For this review, use the dimensioned drawing (mm, ordinates from the lowest corner) and the shaded views. Round coordinates to 2 decimals unless told otherwise and drop trailing zeros. Loops run counter-clockwise (first coordinate to the right, second up) from the corner with the lowest first, then second, coordinate; pieces in that order, holes last.
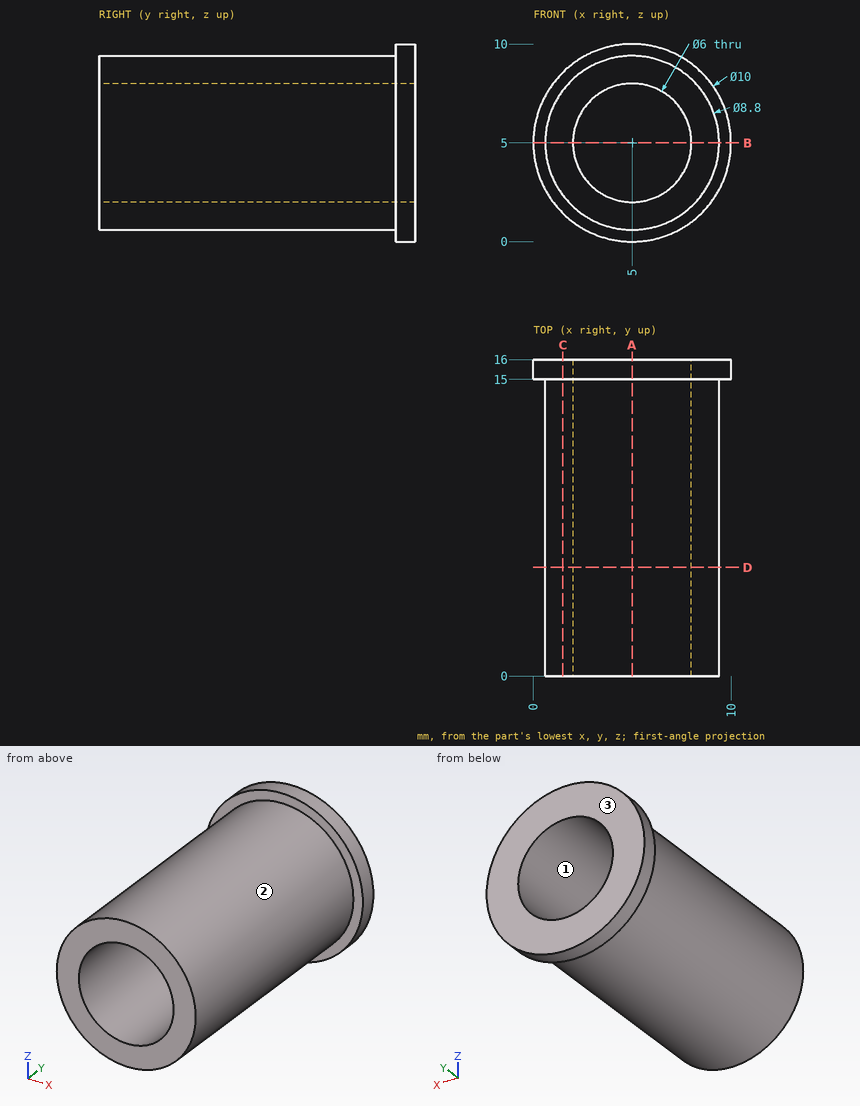
(1) Add section B-B (z = 5). Give the boundary of the cut face in (x, y).
(2) Insertion check: pin 1 Ø1 at (y, z) = (7.5, 1) entering from -X; pin 2 Ø3 at (x, y) = (7.5, 2) entering from +Z; pin 3 Ø4 at (x, y) = (1, 3) entering from +Z. Each pin has a flat end and moves straight along its axis. Give the tip position at first contact, or say it passes through.
(3) Add section D-D (y = 5.5). Give the boundary of the cut face in (x, z), plus the area to 3 significant figures.
(4) Add section C-C (x = 1.5). Give the boundary of the cut face in (y, z).
(5) For L1, parallel to Z at x = 5, y = 8; L2, parallel to Z at x = 3.25, y = 14; L3, parallel to Y at x = 6.75, z = 0.5, list the stretches that pass through material, from the lowest coordinate up.
(6) Add section A-A (x = 5). Give the boundary of the cut face in (y, z), plus the area to 3 significant figures.
(7) The part is to be moulded in two halves that separate along Z. For the marked faces 1, 2 and 3, say which applies: pulls with the +Z half, pulls with the -Z half, needs draft (parallel to the pull), parting line crosses it, or undercut.
Outcome:
1. outline: (0, 15) - (0.6, 15) - (0.6, 0) - (2, 0) - (2, 16) - (0, 16) - close; (8, 0) - (9.4, 0) - (9.4, 15) - (10, 15) - (10, 16) - (8, 16) - close
2. pin 1: stops at x = 2.33
2. pin 2: stops at z = 9.28
2. pin 3: stops at z = 8.92
3. outline: circle Ø8.8 at (5, 5); hole circle Ø6 at (5, 5)
3. area: 32.5 mm2
4. outline: (0, 2.33) - (15, 2.33) - (15, 1.43) - (16, 1.43) - (16, 8.57) - (15, 8.57) - (15, 7.67) - (0, 7.67) - close
5. L1: z = 0.6 to 2, 8 to 9.4
5. L2: z = 0.96 to 2.56, 7.44 to 9.04
5. L3: y = 15 to 16
6. outline: (0, 0.6) - (15, 0.6) - (15, 0) - (16, 0) - (16, 2) - (0, 2) - close; (0, 8) - (16, 8) - (16, 10) - (15, 10) - (15, 9.4) - (0, 9.4) - close
6. area: 46.0 mm2
7. face 1: undercut
7. face 2: parting line crosses it
7. face 3: needs draft
